The figure shows three views and two pictorial views of one solid part (mm, origin at its lowest corner). Answer the questions. A direction names the side the tool comes from. Give positions to 0.01 mm unless a question says otherwise; leave off trailing zeros. Order: outer loops, then holes, each group sorted by start corner. A loop starts at its lowest first (then second) coordinate and runs counter-clockwise, first axis right, second up. Notation, with made-up numbers: M 74.5,46 L 79.5,46 A17 ccw 79.5,52 Z; hole C 43,-40 d5. An arc over 180 degrees is marked long. One line per item, written item: value. Start each with the question number.
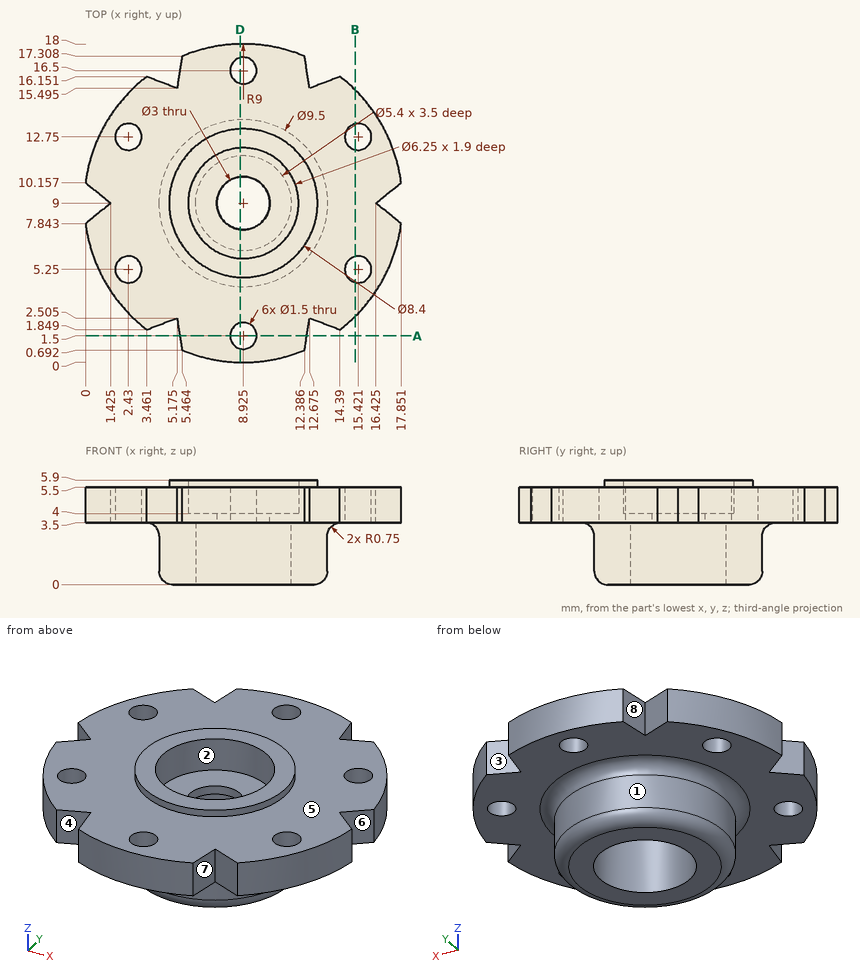
Q1. Find section B-B, the plane x = 15.25. Give the vertices of the cut face in (y, z).
Q2. A tool of negligible diameter and unlimited length cuts with its end or side. For the marked faces 1, 2, 3 and 4, from which of +Z, -Z, +X, -X, +Y, -Y can it reach the whole face along a straight path? Write none if from no direction.
Q3. Find section A-A, the plane y = 1.5. Give the vertices of the cut face in (x, z) (1 decimal).
Q4. Consider probe 1 along Z at (x, y) = (9.75, 2.5); probe 2 along Y at (x, z) = (8.5, 4.7) (1 decimal); probe 3 along Y at (x, z) = (12.5, 2.6) (1 decimal). Determine where each line is inside the solid, lowest interval first.
Q5. Determine the mould class of the marked faces 5, 6, 7 and 8 for opening direction Y: released by +Y, released by -Y, zero draft, split by the parting line, or undercut.
Q6. Each of these flat-tipped pins is pushed along its axis until it touches: pin 1 (2 mm diameter, centred on x = 2.5, y = 13.5, fed in from -Z); pin 2 (2.5 mm diameter, centred on x = 15.42, y = 5.25, fed in from +Z); pin 3 (5.5 mm diameter, centred on x = 8.93, y = 9, fed in from +Z). Where does it stop, or does it pass through?
Q7. Find section D-D, the plane x = 8.75. State how many separate pieces and enclosed holes the cut face has.
Evaluation:
1. outline: M 2.6,3.5 L 4.52,3.5 L 4.52,5.5 L 2.6,5.5 Z; M 5.98,3.5 L 12.02,3.5 L 12.02,5.5 L 5.98,5.5 Z; M 13.48,3.5 L 15.4,3.5 L 15.4,5.5 L 13.48,5.5 Z
2. face 1: -Z
2. face 2: +Z
2. face 3: +Z, -Z, +Y
2. face 4: +Z, -Z, -Y
3. outline: M 5.3,3.5 L 8.2,3.5 L 8.2,5.5 L 5.3,5.5 Z; M 9.7,3.5 L 12.5,3.5 L 12.5,5.5 L 9.7,5.5 Z
4. probe 1: 3.5 to 5.5
4. probe 2: 0 to 0.9, 2.1 to 5.9, 12.1 to 15.9, 17.1 to 18
4. probe 3: 5.9 to 12.1
5. face 5: zero draft
5. face 6: undercut
5. face 7: released by -Y
5. face 8: released by +Y
6. pin 1: z = 3.5
6. pin 2: z = 5.5
6. pin 3: z = 4
7. separate pieces: 4
7. enclosed holes: 0
